Part model, mm, in its own coordinate system. A direction names the side the tool comes from. Give positions to 0.01 mm unless a question says otherwise; leave off trailing zeros. Order: outer loops, then holes, each group sorted by start corner. A loop starts at its lowest first (then second) coordinate and runs counter-clockwise, first axis right, second up. Notation, with made-up numbers: (50, -11.75) - (86, -11.75) arc R22 cw to (86, -5.75) - close; hole circle Ø1 at (18.25, -29.5). An arc over 180 degrees is marked (long way). Use one line per item in the form item = value. Start each with the question number.
1. Band-saw the part on C-C, the plane y = 73.5. State how many separate pieces and enclosed holes the cut face has, plus the area to 3 significant figures.
2. Pin check, flat tips, straight feed: P1, Ø4, axis at y = 55, z = -59.5, coming from the -X side; P2, Ø3, axis at x = 6, z = 8.5, coming from the +Y side; P3, Ø4, axis at y = 1, z = -24.5, coming from the +X side; P4, Ø4, axis at y = 24.5, z = -54, coming from the -X side. Stop position of each tip, or through.
3. Band-saw the part on D-D, the plane z = -38. List the corners of the cut face in (x, y), plus the area to 3 significant figures.
4. Tool access for faces 1 (the face through (-70, 2.5, -42)), 2 (the face through (75, 16, -73)): list every direction of +Z, -Z, +X, -X, +Y, -Y with a clear straight run to the whole face (end or side of a thin tool).
5. Pull direction Y, two halves, no side cores. Call faces 3 (the face through (5, 61, -70)), 4 (the face through (55.73, -54.57, -56.9)): +Y half, -Y half, draft (parallel to the pull), parting line (faces both ways), or undercut.
6. Band-saw the part on A-A, the plane z = -60.5. List the corners of the cut face in (x, y), plus the area to 3 significant figures.
7. Drill centre lines: line 1 (Y direction, x = -1.5, z = 16.5); line 2 (X direction, y = 0, z = 8); line 3 (X direction, y = 0, z = -65.6). Where is each one in solid material? Low to high.
8. Band-saw the part on B-B, the plane z = -11. List the corners of the cut face in (x, y).
from build123d import *

# Parameters (mm, degrees)
CUT_EXTRUDE7_DEPTH   = 14
BOSS_EXTRUDE10_START = 5
BOSS_EXTRUDE10_DEPTH = 5
BOSS_EXTRUDE11_DEPTH = 2.5
CIRPATTERN1_COUNT    = 4


with BuildPart() as part:
    # Sketch10 → Revolve2 (revolve)
    with BuildSketch(Plane(origin=(0, 0, 0), x_dir=(1, 0, 0), z_dir=(0, 1, 0))):
        Polygon((68, 0), (85, 50), (82, 50), (82, 70), (60, 70), (60, 64), (78, 64), (78, 50), (78.018901629, 45), (65, 6.709112855), (65, -20), (68, -20), align=None)
    revolve(axis=Axis((0, 0, 0), (0, 0, -1)))

    # Sketch19 → Cut-Extrude7 (cut)
    with BuildSketch(Plane(origin=(0, 0, -50), x_dir=(-1, 0, 0), z_dir=(0, 0, -1))):
        with BuildLine():
            Line((-75.342214451, 20.187885518), (-79.205917756, 21.223161698))
            ThreePointArc((-79.205917756, 21.223161698), (-72.734888321, 37.863386285), (-62.815644336, 52.708583994))
            Line((-62.815644336, 52.708583994), (-59.751466563, 50.137433556))
            ThreePointArc((-59.751466563, 50.137433556), (-69.186844988, 36.016391832), (-75.342214451, 20.187885518))
        make_face()
        with BuildLine():
            Line((59.751466563, 50.137433556), (62.815644336, 52.708583994))
            ThreePointArc((62.815644336, 52.708583994), (72.734888321, 37.863386285), (79.205917756, 21.223161698))
            Line((79.205917756, 21.223161698), (75.342214451, 20.187885518))
            ThreePointArc((75.342214451, 20.187885518), (69.186844988, 36.016391832), (59.751466563, 50.137433556))
        make_face()
    extrude(amount=CUT_EXTRUDE7_DEPTH, mode=Mode.SUBTRACT)

    # Sketch29 → Boss-Extrude10 (add)
    with BuildSketch(Plane(origin=(0, 0, -70), x_dir=(-1, 0, 0), z_dir=(0, 0, -1)).offset(BOSS_EXTRUDE10_START)):
        with BuildLine():
            Line((-75, 0), (-75, 33.151168909))
            ThreePointArc((-75, 33.151168909), (0, -82), (75, 33.151168909))
            Line((75, 33.151168909), (75, 0))
            ThreePointArc((75, 0), (0, -75), (-75, 0))
        make_face()
    extrude(amount=-BOSS_EXTRUDE10_DEPTH)

    # Sketch37 → Boss-Extrude11 (add, symmetric)
    with BuildSketch(Plane(origin=(0, 0, 0), x_dir=(1, 0, 0), z_dir=(0, 1, 0))):
        Polygon((-65, 6.709112855), (-65, 70), (-78, 64), (-78.018901629, 45), align=None)
    boss_extrude11 = extrude(amount=BOSS_EXTRUDE11_DEPTH, both=True)

    # CirPattern1: Boss-Extrude11 ×4 about axis
    cirpattern1_axis = Axis((0, 0, 0), (0, 0, 1))
    for i in range(1, CIRPATTERN1_COUNT):
        add(boss_extrude11.rotate(cirpattern1_axis, i * 360 / CIRPATTERN1_COUNT))


solid = part.part
From the geometry:
q1.separate_pieces = 1
q1.enclosed_holes = 2
q1.area = 2,060 mm²
q2.P1 = -62.57
q2.P2 = 67.85
q2.P3 = 77
q2.P4 = through
q3.outline = circle Ø161.84 at (0, 0); hole (-75.6, -2.5) arc R75.64 ccw to (-2.5, -75.6) - (-2.5, -65) - (2.5, -65) - (2.5, -75.6) arc R75.64 ccw to (75.6, -2.5) - (65, -2.5) - (65, 2.5) - (75.6, 2.5) arc R75.64 ccw to (2.5, 75.6) - (2.5, 65) - (-2.5, 65) - (-2.5, 75.6) arc R75.64 ccw to (-75.6, 2.5) - (-65, 2.5) - (-65, -2.5) - close
q3.area = 2,810 mm²
q4.face_1 = none
q4.face_2 = -Z, +Y
q5.face_3 = draft
q5.face_4 = undercut
q6.outline = (-79.21, 21.22) arc R82 ccw (long way) to (79.21, 21.22) - (75.34, 20.19) arc R78 cw to (77.96, 2.5) - (65, 2.5) - (65, -2.5) - (77.96, -2.5) arc R78 cw to (2.5, -77.96) - (2.5, -65) - (-2.5, -65) - (-2.5, -77.96) arc R78 cw to (-77.96, -2.5) - (-65, -2.5) - (-65, 2.5) - (-77.96, 2.5) arc R78 cw to (-75.34, 20.19) - close; (-62.82, 52.71) - (-59.75, 50.14) arc R78 cw to (-2.5, 77.96) - (-2.5, 65) - (2.5, 65) - (2.5, 77.96) arc R78 cw to (59.75, 50.14) - (62.82, 52.71) arc R82 ccw to start
q6.area = 1,990 mm²
q7.line_1 = -67.98 to -64.98, 64.98 to 67.98
q7.line_2 = -68 to -65, 65 to 68
q7.line_3 = -82 to -60, 60 to 82
q8.outline = circle Ø143.48 at (0, 0); hole (-66.41, -2.5) arc R66.46 ccw to (-2.5, -66.41) - (-2.5, -65) - (2.5, -65) - (2.5, -66.41) arc R66.46 ccw to (66.41, -2.5) - (65, -2.5) - (65, 2.5) - (66.41, 2.5) arc R66.46 ccw to (2.5, 66.41) - (2.5, 65) - (-2.5, 65) - (-2.5, 66.41) arc R66.46 ccw to (-66.41, 2.5) - (-65, 2.5) - (-65, -2.5) - close
